from build123d import *

# Parameters (mm, degrees)
CROQUIS1_R              = 2
CROQUIS1_W              = 53.3
CROQUIS1_H              = 20.15
SALIENTE_EXTRUIR1_DEPTH = 8
CROQUIS2_W              = 8
CROQUIS2_H              = 20.15
CROQUIS2_W_2            = 5
SALIENTE_EXTRUIR2_DEPTH = 8
CROQUIS2_4_W            = 5
CROQUIS2_4_H            = 20.15
SALIENTE_EXTRUIR3_DEPTH = 10
CROQUIS2_5_W            = 8
CROQUIS2_5_H            = 20.15
SALIENTE_EXTRUIR4_DEPTH = 32
CROQUIS4_R              = 2
CORTAR_EXTRUIR1_DEPTH   = 32
CROQUIS4_2_R            = 2
CORTAR_EXTRUIR2_DEPTH   = 74
CROQUIS5_R              = 2.65
CORTAR_EXTRUIR3_DEPTH   = 35
CORTAR_EXTRUIR4_DEPTH   = 16
CORTAR_EXTRUIR5_DEPTH   = 16


with BuildPart() as part:
    # Croquis1 → Saliente-Extruir1 (new body)
    with BuildSketch(Plane(origin=(0, 0, 0), x_dir=(1, 0, 0), z_dir=(0, 1, 0))):
        Polygon((154, 0), (156.998132752, 2.998132752), (156.998132752, 6.998132752), (154.446539538, 11.574918968), (101.665094886, 44.198861104), (97.772883017, 48.458390041), (88.347282669, 67.313746258), (84.009081739, 69.99516616), (26.841381739, 69.99516616), (-2.995601596, 10.334082852), (-2.995601596, 3.004082852), (0, 0), align=None)
        with Locations((2, 4.998132752)):
            Circle(CROQUIS1_R, mode=Mode.SUBTRACT)
        with Locations((57, 4.998132752)):
            Circle(CROQUIS1_R, mode=Mode.SUBTRACT)
        with Locations((114, 4.998132752)):
            Circle(CROQUIS1_R, mode=Mode.SUBTRACT)
        with Locations((152, 4.998132752)):
            Circle(CROQUIS1_R, mode=Mode.SUBTRACT)
        with Locations((55.5, 50.075)):
            Rectangle(CROQUIS1_W, CROQUIS1_H, mode=Mode.SUBTRACT)
    extrude(amount=SALIENTE_EXTRUIR1_DEPTH)

    # Croquis2 → Saliente-Extruir2 (add)
    with BuildSketch(Plane(origin=(0, 8, 0), x_dir=(1, 0, 0), z_dir=(0, 1, 0))):
        with Locations((32.85, 50.075)):
            Rectangle(CROQUIS2_W, CROQUIS2_H)
        with Locations((79.65, 50.075)):
            Rectangle(CROQUIS2_W_2, CROQUIS2_H)
    extrude(amount=-SALIENTE_EXTRUIR2_DEPTH)

    # Croquis2_4 → Saliente-Extruir3 (add)
    with BuildSketch(Plane(origin=(0, 8, 0), x_dir=(1, 0, 0), z_dir=(0, 1, 0))):
        with Locations((79.65, 50.075)):
            Rectangle(CROQUIS2_4_W, CROQUIS2_4_H)
    extrude(amount=SALIENTE_EXTRUIR3_DEPTH)

    # Croquis2_5 → Saliente-Extruir4 (add)
    with BuildSketch(Plane(origin=(0, 8, 0), x_dir=(1, 0, 0), z_dir=(0, 1, 0))):
        with Locations((32.85, 50.075)):
            Rectangle(CROQUIS2_5_W, CROQUIS2_5_H)
    extrude(amount=SALIENTE_EXTRUIR4_DEPTH)

    # Croquis4 → Cortar-Extruir1 (cut)
    with BuildSketch(Plane.ZY.offset(-77.15)):
        with Locations((-50.075, 13)):
            Circle(CROQUIS4_R)
    extrude(amount=-CORTAR_EXTRUIR1_DEPTH, mode=Mode.SUBTRACT)

    # Croquis4_2 → Cortar-Extruir2 (cut)
    with BuildSketch(Plane.ZY.offset(-77.15)):
        with Locations((-50.075, 13)):
            Circle(CROQUIS4_2_R)
    extrude(amount=CORTAR_EXTRUIR2_DEPTH, mode=Mode.SUBTRACT)

    # Croquis5 → Cortar-Extruir3 (cut)
    with BuildSketch(Plane(origin=(36.85, 0, 0), x_dir=(0, 0, -1), z_dir=(1, 0, 0))):
        with Locations((50.08, 30)):
            Circle(CROQUIS5_R)
    extrude(amount=-CORTAR_EXTRUIR3_DEPTH, mode=Mode.SUBTRACT)

    # Croquis6 → Cortar-Extruir4 (cut)
    with BuildSketch(Plane(origin=(82.15, 0, 0), x_dir=(0, 0, -1), z_dir=(1, 0, 0))):
        with BuildLine():
            Line((40, 17), (40, 18))
            Line((40, 18), (41, 18))
            ThreePointArc((41, 18), (40.292893219, 17.707106781), (40, 17))
        make_face()
        with BuildLine():
            Line((59.15, 18), (60.15, 18))
            Line((60.15, 18), (60.15, 17))
            ThreePointArc((60.15, 17), (59.857106781, 17.707106781), (59.15, 18))
        make_face()
    extrude(amount=-CORTAR_EXTRUIR4_DEPTH, mode=Mode.SUBTRACT)

    # Croquis7 → Cortar-Extruir5 (cut)
    with BuildSketch(Plane(origin=(36.85, 0, 0), x_dir=(0, 0, -1), z_dir=(1, 0, 0))):
        with BuildLine():
            Line((40, 35), (40, 40))
            Line((40, 40), (45, 40))
            ThreePointArc((45, 40), (41.464466094, 38.535533906), (40, 35))
        make_face()
        with BuildLine():
            Line((55.15, 40), (60.15, 40))
            Line((60.15, 40), (60.15, 35))
            ThreePointArc((60.15, 35), (58.685533906, 38.535533906), (55.15, 40))
        make_face()
    extrude(amount=-CORTAR_EXTRUIR5_DEPTH, mode=Mode.SUBTRACT)


solid = part.part
Design review of the part built by this model. Coordinates are the model's own, in mm. A direction names the side the tool comes from. Round coordinates to 2 decimals unless told otherwise and drop trailing zeros. Write each loop counter-clockwise with the first axis right and the second up, starting at its lowest first coordinate (ties: lowest second). Pieces come first, ordered by that corner, then holes. Notation, with made-up numbers: (-16.75, 23) -> (36.25, 23) arc R15 ccw to (36.25, 46) -> close; hole circle Ø8 at (-6.75, 73). An arc over 180 degrees is marked (long way). One line per item, written item: value. Start each with the question number.
Q1. Add section C-C (y = 4.5). Give the boundary of the cut face in (x, z).
Q2. To check wall thickness, follow probe 1 along Z at (x, y) = (57, 5); probe 2 along Z at (x, y) = (47, 4.5); probe 3 along Y at (x, z) = (88, -35.5). State the ranges of each line that lie inside material, in increasing order.
Q3. Tool access review of faces 1 (the face through (80, 12, -40)), 2 (the face through (156.998, 4, -5)), 3 (the face through (82.15, 10.7, -49.9)): name each direction out of +Z, -Z, +X, -X, +Y, -Y from which nothing blocks a thin tool from reaching the whole face with its end or side.
Q4. Insertion check: P1, Ø5.5, axis at y = 7.5, z = -51, coming from the -X side; P2, Ø5, axis at x = 114, z = -5, coming from the +Y side; P3, Ø16, axis at y = 19.5, z = -50, coming from the -X side; P4, Ø12, axis at x = 67, z = -51.5, coming from the +Y side. Each pin has a flat end and moves straight along its axis. Give the tip position at first contact, or say it passes through.
Q5. Add section B-B (y = 30). Give the boundary of the cut face in (x, z), then the cut area to 3 significant figures.
Q6. Add section A-A (x = 68). Give the boundary of the cut face in (y, z), then the cut area to 3 significant figures.
Q7. Add section D-D (x = 95). Give the boundary of the cut face in (y, z), then the cut area to 3 significant figures.
Q8. The part is to be moulded in two halves that separate along Z. For faces 4 (the face through (112, 4, -5)), 5 (the face through (-2.996, 4, -7)), 6 (the face through (93.13, 3.94, -57.75)), say which applies: pulls with the +Z half, pulls with the -Z half, needs draft (parallel to the pull), parting line crosses it, or undercut.
Response:
1. outline: (-3, -10.33) -> (26.84, -70) -> (84.01, -70) -> (88.35, -67.31) -> (97.77, -48.46) -> (101.67, -44.2) -> (154.45, -11.57) -> (157, -7) -> (157, -3) -> (154, 0) -> (0, 0) -> (-3, -3) -> close; hole circle Ø4 at (2, -5); hole (36.85, -60.15) -> (77.15, -60.15) -> (77.15, -40) -> (36.85, -40) -> close; hole circle Ø4 at (57, -5); hole circle Ø4 at (114, -5); hole circle Ø4 at (152, -5)
2. probe 1: z = -70 to -60.15, -40 to -7, -3 to 0
2. probe 2: z = -70 to -60.15, -40 to 0
2. probe 3: y = 0 to 8
3. face 1: +Z, +X, -X, +Y
3. face 2: +Z, -Z, +X, +Y, -Y
3. face 3: +Z, -Z, +X, +Y
4. P1: stops at x = 15.97
4. P2: stops at y = 8
4. P3: stops at x = 28.85
4. P4: passes through
5. outline: (28.85, -60.15) -> (36.85, -60.15) -> (36.85, -52.73) -> (28.85, -52.73) -> close; (28.85, -47.43) -> (36.85, -47.43) -> (36.85, -40) -> (28.85, -40) -> close
5. area: 119 mm^2
6. outline: (0, -70) -> (8, -70) -> (8, -60.15) -> (0, -60.15) -> close; (0, -40) -> (8, -40) -> (8, 0) -> (0, 0) -> close
6. area: 399 mm^2
7. outline: (0, -54.01) -> (8, -54.01) -> (8, 0) -> (0, 0) -> close
7. area: 432 mm^2
8. face 4: undercut
8. face 5: needs draft
8. face 6: pulls with the -Z half
